from build123d import *

# Parameters (mm, degrees)
BOSS_EXTRUDE1_DEPTH = 140
SKETCH2_R           = 18.75
CUT_EXTRUDE1_DEPTH  = 147.650093761


with BuildPart() as part:
    # Sketch1 → Boss-Extrude1 (new body)
    with BuildSketch(Plane(origin=(0, 0, 0), x_dir=(0, 0, -1), z_dir=(1, 0, 0))):
        Polygon((0.16, 27.66), (5, 27.66), (5, 42.5), (-5, 42.5), (-5, -42.5), (5, -42.5), (5, -27.66), (-0.16, -27.66), (-0.16, -25.66), (-3.16, -25.66), (-3.16, -19.34), (-0.16, -19.34), (-0.16, -12.650615569), (5, -12.650615569), (5, 12.650615569), (-0.16, 12.650615569), (-0.16, 19.34), (-3.16, 19.34), (-3.16, 25.66), (0.16, 25.66), align=None)
    extrude(amount=BOSS_EXTRUDE1_DEPTH)

    # Sketch2 → Cut-Extrude1 (cut, through all)
    with BuildSketch(Plane.XY.offset(5)):
        with Locations((70, 0)):
            Circle(SKETCH2_R)
    extrude(amount=-CUT_EXTRUDE1_DEPTH, mode=Mode.SUBTRACT)


solid = part.part
Verification items for the finished model (mm, model axes). A direction names the side the tool comes from. Coordinates: 2 decimals unless noted, no trailing zeros. Order: outer loops, then holes, each group sorted by start corner. A loop starts at its lowest first (then second) coordinate and runs counter-clockwise, first axis right, second up. Notation, with made-up numbers: M 13,45.5 L 50,45.5 A30 ccw 50,81.5 Z; hole C -4,75 d8. An arc over 180 degrees is marked long. Write each question's results on one line, items separated by ' | '.
1) Scan lines: line 1 along Y through (x, z) = (98, -4.5); line 2 along Y through (x, z) = (25.5, 1.75); line 3 along Y through (x, z) = (70, 1.5). Record each from-to range of solid material in increasing order. Write a range as [from, to].
Solved:
line 1: y = [-42.5, -27.66], [-12.65, 12.65], [27.66, 42.5] | line 2: y = [-42.5, -25.66], [-19.34, 19.34], [25.66, 42.5] | line 3: y = [-42.5, -25.66], [-19.34, -18.75], [18.75, 19.34], [25.66, 42.5]
2) Section check B-B on y = 0. Record the cut outline in (x, z).
Solved:
outline: M 0,-5 L 51.25,-5 L 51.25,5 L 0,5 Z; M 88.75,-5 L 140,-5 L 140,5 L 88.75,5 Z
3) Section check A-A on x = 70. Record the cut outline in (y, z).
Solved:
outline: M -42.5,-5 L -27.66,-5 L -27.66,0.16 L -25.66,0.16 L -25.66,3.16 L -19.34,3.16 L -19.34,0.16 L -18.75,0.16 L -18.75,5 L -42.5,5 Z; M 18.75,0.16 L 19.34,0.16 L 19.34,3.16 L 25.66,3.16 L 25.66,-0.16 L 27.66,-0.16 L 27.66,-5 L 42.5,-5 L 42.5,5 L 18.75,5 Z
4) Gauge pin test, flat ends, axial feed: pin 1 Ø1.9 at (x, y) = (65.5, -22.5) entering from -Z; pin 2 Ø0.6 at (x, y) = (41.5, -26.5) entering from -Z. Record the tip position at first contact, or that the pin passes through.
Solved:
pin 1: stops at z = 3.16 | pin 2: stops at z = 0.16
5) Release check for a two-part mould opening along Y. For faces 1 (the face through (69, 19.34, 2)), 2 (the face through (69, 19, 0.16)), 3 (the face through (53, 10, 5)), 4 (the face through (69, 42.5, 0)) record: pulls with the +Y half, pulls with the -Y half, needs draft (parallel to the pull), parting line crosses it, or undercut.
Solved:
face 1: undercut | face 2: undercut | face 3: needs draft | face 4: pulls with the +Y half
6) Section check D-D on y = 15. Record the cut outline in (x, z), plus the area to 3 significant figures.
Solved:
outline: M 0,0.16 L 58.75,0.16 L 58.75,5 L 0,5 Z; M 81.25,0.16 L 140,0.16 L 140,5 L 81.25,5 Z | area: 569 mm²
7) Section check C-C on z = -3.5. Record the cut outline in (x, y), plus the area to 3 significant figures.
Solved:
outline: M 0,-42.5 L 140,-42.5 L 140,-27.66 L 0,-27.66 Z; M 0,-12.65 L 56.16,-12.65 A18.75 cw 56.16,12.65 L 0,12.65 Z; M 0,27.66 L 140,27.66 L 140,42.5 L 0,42.5 Z; M 83.84,-12.65 L 140,-12.65 L 140,12.65 L 83.84,12.65 A18.75 cw Z | area: 6,830 mm²
8) Access from +Z, -Z, +X, -X, +Y, -Y to the whole of each face (thin tool, end or side, straight path). Record for faces 5 (the face through (69, 22, 3.16)), 6 (the face through (69, -35, -5)).
Solved:
face 5: -Z, +X, -X | face 6: -Z, +X, -X, +Y, -Y
